from build123d import *

# Parameters (mm, degrees)
F0_W      = 101.5
F0_H      = 85
F1_DEPTH  = 15.875
F2_R      = 16.25
F3_DEPTH  = 25
F4_W      = 101.5
F4_H      = 85
F5_DEPTH  = 5.875
F7_DEPTH  = 12
F8_W      = 78.5
F8_H      = 10
F9_DEPTH  = 3.5
F10_W     = 78.5
F10_H     = 10
F11_DEPTH = 3.5
F12_W     = 78.5
F12_H     = 3
F13_DEPTH = 25
F14_W     = 78.5
F14_H     = 17.569206
F15_DEPTH = 200
F16_W     = 78.5
F16_H     = 75
F17_DEPTH = 6.125
F18_R     = 1.5
F18_W     = 66.5
F18_H     = 3
F19_DEPTH = 2
F20_R     = 1.5
F20_W     = 66.5
F20_H     = 3
F21_DEPTH = 2
F22_R     = 2.5
F23_DEPTH = 10
F24_R     = 2.5
F25_DEPTH = 10
F26_R     = 2.5
F27_DEPTH = 5
F28_R     = 2.5
F29_DEPTH = 5
F30_W     = 91.57778
F30_H     = 6.951566
F30_W_2   = 93.047712
F30_H_2   = 9.166792
F31_DEPTH = 5.875


with BuildPart() as f1:
    # F0 (on Front) → F1 (new body)
    with BuildSketch(Plane.XZ):
        Rectangle(F0_W, F0_H)
    extrude(amount=F1_DEPTH)

    # F2 (on face) → F3 (cut)
    with BuildSketch(Plane.XZ.offset(15.875)):
        Circle(F2_R)
    extrude(amount=-F3_DEPTH, mode=Mode.SUBTRACT)

    # F4 (on face) → F5 (cut)
    with BuildSketch(Plane(origin=(0, 0, 0), x_dir=(-1, 0, 0), z_dir=(0, 1, 0))):
        Rectangle(F4_W, F4_H)
        with BuildLine():
            Line((-45.75, -31), (-45.75, 31))
            ThreePointArc((-45.75, 31), (-43.846194, 35.596194), (-39.25, 37.5))
            Line((-39.25, 37.5), (39.25, 37.5))
            ThreePointArc((39.25, 37.5), (43.846194, 35.596194), (45.75, 31))
            Line((45.75, 31), (45.75, -31))
            ThreePointArc((45.75, -31), (43.846194, -35.596194), (39.25, -37.5))
            Line((39.25, -37.5), (-39.25, -37.5))
            ThreePointArc((-39.25, -37.5), (-43.846194, -35.596194), (-45.75, -31))
        make_face(mode=Mode.SUBTRACT)
    extrude(amount=-F5_DEPTH, mode=Mode.SUBTRACT)

    # F6 (on face) → F7 (cut)
    with BuildSketch(Plane(origin=(0, 0, 0), x_dir=(-1, 0, 0), z_dir=(0, 1, 0))):
        with BuildLine():
            ThreePointArc((-36.25, 34.5), (-40.846194, 32.596194), (-42.75, 28))
            Line((-42.75, 28), (-42.75, -28))
            ThreePointArc((-42.75, -28), (-40.846194, -32.596194), (-36.25, -34.5))
            Line((-36.25, -34.5), (36.25, -34.5))
            ThreePointArc((36.25, -34.5), (40.846194, -32.596194), (42.75, -28))
            Line((42.75, -28), (42.75, 28))
            ThreePointArc((42.75, 28), (40.846194, 32.596194), (36.25, 34.5))
            Line((36.25, 34.5), (-36.25, 34.5))
        make_face()
    extrude(amount=-F7_DEPTH, mode=Mode.SUBTRACT)

    # F8 (on face) → F9 (cut)
    with BuildSketch(Plane.XY.offset(42.5)):
        with Locations((0, -10.875)):
            Rectangle(F8_W, F8_H)
    extrude(amount=-F9_DEPTH, mode=Mode.SUBTRACT)

    # F10 (on face) → F11 (cut)
    with BuildSketch(Plane(origin=(0, 0, -42.5), x_dir=(1, 0, 0), z_dir=(0, 0, -1))):
        with Locations((0, 10.875)):
            Rectangle(F10_W, F10_H)
    extrude(amount=-F11_DEPTH, mode=Mode.SUBTRACT)

    # F12 (on face) → F13 (cut)
    with BuildSketch(Plane.XZ.offset(15.875)):
        with Locations((0, 36)):
            Rectangle(F12_W, F12_H)
        with Locations((0, -36)):
            Rectangle(F12_W, F12_H)
    extrude(amount=-F13_DEPTH, mode=Mode.SUBTRACT)

    # F14 (on face) → F15 (cut)
    with BuildSketch(Plane.XY.offset(39)):
        with Locations((0, 2.909603)):
            Rectangle(F14_W, F14_H)
    extrude(amount=-F15_DEPTH, mode=Mode.SUBTRACT)

    # F16 (on face) → F17 (cut)
    with BuildSketch(Plane(origin=(0, -5.875, 0), x_dir=(-1, 0, 0), z_dir=(0, 1, 0))):
        Rectangle(F16_W, F16_H)
    extrude(amount=-F17_DEPTH, mode=Mode.SUBTRACT)

    # F18 (on face) → F19 (cut)
    with BuildSketch(Plane.XY.offset(39)):
        with Locations((-34.75, -10.375)):
            Circle(F18_R)
        with Locations((3, -10.375)):
            Rectangle(F18_W, F18_H)
    extrude(amount=-F19_DEPTH, mode=Mode.SUBTRACT)

    # F20 (on face) → F21 (cut)
    with BuildSketch(Plane(origin=(0, 0, -39), x_dir=(1, 0, 0), z_dir=(0, 0, -1))):
        with Locations((34.75, 10.375)):
            Circle(F20_R)
        with Locations((-3, 10.375)):
            Rectangle(F20_W, F20_H)
    extrude(amount=-F21_DEPTH, mode=Mode.SUBTRACT)

    # F22 (on face) → F23 (cut)
    with BuildSketch(Plane(origin=(0, 0, -42.5), x_dir=(1, 0, 0), z_dir=(0, 0, -1))):
        with Locations((-45, 10.875)):
            Circle(F22_R)
    extrude(amount=-F23_DEPTH, mode=Mode.SUBTRACT)

    # F24 (on face) → F25 (cut)
    with BuildSketch(Plane(origin=(0, 0, -42.5), x_dir=(1, 0, 0), z_dir=(0, 0, -1))):
        with Locations((45, 10.875)):
            Circle(F24_R)
    extrude(amount=-F25_DEPTH, mode=Mode.SUBTRACT)

    # F26 (on face) → F27 (cut)
    with BuildSketch(Plane.XY.offset(42.5)):
        with Locations((-45, -10.875)):
            Circle(F26_R)
    extrude(amount=-F27_DEPTH, mode=Mode.SUBTRACT)

    # F28 (on face) → F29 (cut)
    with BuildSketch(Plane.XY.offset(42.5)):
        with Locations((45, -10.875)):
            Circle(F28_R)
    extrude(amount=-F29_DEPTH, mode=Mode.SUBTRACT)

    # F30 (on face) → F31 (cut)
    with BuildSketch(Plane(origin=(0, 0, 0), x_dir=(-1, 0, 0), z_dir=(0, 1, 0))):
        with Locations((0.03889, 34.475783)):
            Rectangle(F30_W, F30_H)
        with Locations((0.773856, -35.583396)):
            Rectangle(F30_W_2, F30_H_2)
    extrude(amount=-F31_DEPTH, mode=Mode.SUBTRACT)


solid = f1.part
Geometry check sheet. Reference: the model listing, model coordinates, mm. A direction names the side the tool comes from. Round coordinates to 2 decimals unless told otherwise and drop trailing zeros. Write each loop counter-clockwise with the first axis right and the second up, starting at its lowest first coordinate (ties: lowest second). Pieces come first, ordered by that corner, then holes.
Item 1: Mould release check, pull along Y, two halves, no side actions. Record for faces 1 (the face through (39.25, -11, -41)), 2 (the face through (47.31, -11.83, 40.03)), 3 (the face through (-35.94, -11.29, 38.26)), 4 (the face through (10, -12, 16)): +Y half, -Y half, draft (parallel to the pull), parting line (faces both ways), or undercut.
Determined:
face 1: draft
face 2: undercut
face 3: undercut
face 4: +Y half
Item 2: Go/stop test with flat-tipped pins: pin 1 Ø1.2 at (x, y) = (-17, -13) entering from -Z; pin 2 Ø4.5 at (y, z) = (-2.5, 5) entering from -X; pin 3 Ø3 at (x, y) = (-11, -13.5) entering from +Z. Record where each tip stops, or that it passes through.
Determined:
pin 1: stops at z = -39
pin 2: stops at x = -45.75
pin 3: stops at z = 39
Item 3: Access from +Z, -Z, +X, -X, +Y, -Y to the whole of each face (thin tool, end or side, straight path). Record for faces 5 (the face through (47.3, -9.9, -37.6)), 6 (the face through (-0.5, -12.1, 37.5)), 7 (the face through (39.25, -11, 36)), 8 (the face through (-42.69, -11.83, 40.03)).
Determined:
face 5: -Z
face 6: +Y, -Y
face 7: +Y
face 8: +Z
Item 4: Section check B-B (z = 9.5). Record the boundary of the cut face in (x, y) (3 decimals).
Determined:
outline: (-50.75, -15.875) - (-13.184, -15.875) - (-13.184, -12) - (-42.75, -12) - (-42.75, 0) - (-45.75, 0) - (-45.75, -5.875) - (-50.75, -5.875) - close; (13.184, -15.875) - (50.75, -15.875) - (50.75, -5.875) - (45.75, -5.875) - (45.75, 0) - (42.75, 0) - (42.75, -12) - (13.184, -12) - close
Item 5: Section check C-C (x = 0). Record the boundary of the cut face in (y, z) (3 decimals).
Determined:
outline: (-15.875, -39) - (-11.875, -39) - (-11.875, -37.5) - (-15.875, -37.5) - close; (-15.875, -34.5) - (-12, -34.5) - (-12, -16.25) - (-15.875, -16.25) - close; (-15.875, 16.25) - (-12, 16.25) - (-12, 34.5) - (-15.875, 34.5) - close; (-15.875, 37.5) - (-11.875, 37.5) - (-11.875, 39) - (-15.875, 39) - close; (-8.875, -39) - (-5.875, -39) - (-5.875, -37.5) - (-8.875, -37.5) - close; (-8.875, 37.5) - (-5.875, 37.5) - (-5.875, 39) - (-8.875, 39) - close
Item 6: Section check A-A (x = 34.75). Record the boundary of the cut face in (y, z) (3 decimals), plus the area to 3 significant figures.
Determined:
outline: (-15.875, -39) - (-11.875, -39) - (-11.875, -37.5) - (-15.875, -37.5) - close; (-15.875, -34.5) - (-12, -34.5) - (-12, 34.5) - (-15.875, 34.5) - close; (-15.875, 37.5) - (-11.875, 37.5) - (-11.875, 39) - (-15.875, 39) - close; (-8.875, -39) - (-5.875, -39) - (-5.875, -37.5) - (-8.875, -37.5) - close; (-8.875, 37.5) - (-5.875, 37.5) - (-5.875, 39) - (-8.875, 39) - close
area: 288 mm2
Item 7: Material ranges on line 1 along Z through (x, y) = (26, -13); line 2 along Z through (x, y) = (0, -14.95); line 3 along Z through (x, y) = (-11.5, -7.75), recorded low to high.
Determined:
line 1: z = -39 to -37.5, -34.5 to 34.5, 37.5 to 39
line 2: z = -39 to -37.5, -34.5 to -16.25, 16.25 to 34.5, 37.5 to 39
line 3: z = -39 to -37.5, 37.5 to 39
Item 8: Section check D-D (x = 11.5). Record the boundary of the cut face in (y, z) (3 decimals), plus the area to 3 significant figures.
Determined:
outline: (-15.875, -39) - (-11.875, -39) - (-11.875, -37.5) - (-15.875, -37.5) - close; (-15.875, -34.5) - (-12, -34.5) - (-12, -11.481) - (-15.875, -11.481) - close; (-15.875, 11.481) - (-12, 11.481) - (-12, 34.5) - (-15.875, 34.5) - close; (-15.875, 37.5) - (-11.875, 37.5) - (-11.875, 39) - (-15.875, 39) - close; (-8.875, -39) - (-5.875, -39) - (-5.875, -37.5) - (-8.875, -37.5) - close; (-8.875, 37.5) - (-5.875, 37.5) - (-5.875, 39) - (-8.875, 39) - close
area: 199 mm2
